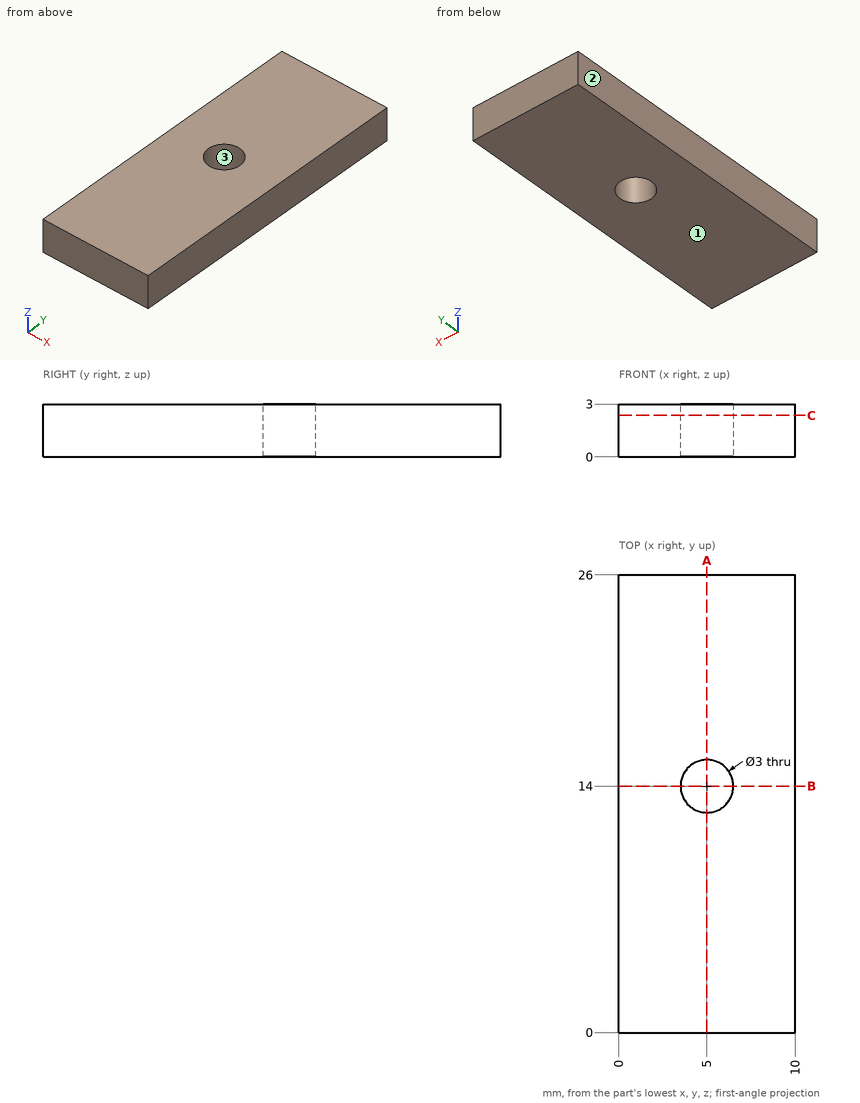
Geometry check sheet. Reference: drawing and pictorial views, mm from the part's lowest x, y, z. Round coordinates to 2 decimals unless told otherwise and drop trailing zeros. Order: outer loops, then holes, each group sorted by start corner. A loop starts at its lowest first (then second) coordinate and runs counter-clockwise, first axis right, second up. Notation, with made-up numbers: (37, 4) - (78, 4) arc R24 ccw to (78, 24) - close; hole circle Ø2 at (-29, -32.5). An arc over 180 degrees is marked (long way). Write item = value, one per line.
Q1. Section check C-C (z = 2.35). Record the boundary of the cut face in (x, y), and give its area (3 significant figures).
Computed:
outline = (0, 0) - (10, 0) - (10, 26) - (0, 26) - close; hole circle Ø3 at (5, 14)
area = 253 mm^2
Q2. Section check B-B (y = 14). Record the boundary of the cut face in (x, z), and give its area (3 significant figures).
Computed:
outline = (0, 0) - (3.5, 0) - (3.5, 3) - (0, 3) - close; (6.5, 0) - (10, 0) - (10, 3) - (6.5, 3) - close
area = 21.0 mm^2
Q3. Section check A-A (x = 5). Record the boundary of the cut face in (y, z), and give its area (3 significant figures).
Computed:
outline = (0, 0) - (12.5, 0) - (12.5, 3) - (0, 3) - close; (15.5, 0) - (26, 0) - (26, 3) - (15.5, 3) - close
area = 69.0 mm^2
Q4. Draft check along X on the marked faces 1, 2 and 3. Enter one of: pulls with the +X half, pulls with the -X half, needs draft (parallel to the pull), parting line crosses it, or undercut.
Computed:
face_1 = needs draft
face_2 = pulls with the -X half
face_3 = undercut
Q5. Thickness scan on line 1 along Y through (x, z) = (5, 0.75); line 2 along X through (y, z) = (13.5, 0.95); line 3 along X through (y, z) = (15.25, 1.95). Record the ranges inside material, lowest first.
Computed:
line_1 = 0 to 12.5, 15.5 to 26
line_2 = 0 to 3.59, 6.41 to 10
line_3 = 0 to 4.17, 5.83 to 10
